Answer from the drawing. Dimensions are ordinates in mm from the lowest x, y and z of the part. A direction names the side the tool comes from. Give positions to 0.01 mm unless a question says otherwise; leave off trailing zeros. Order: outer loops, then holes, each group sorted by start corner. A loop starts at its lowest first (then second) coordinate and runs counter-clockwise, first axis right, second up.
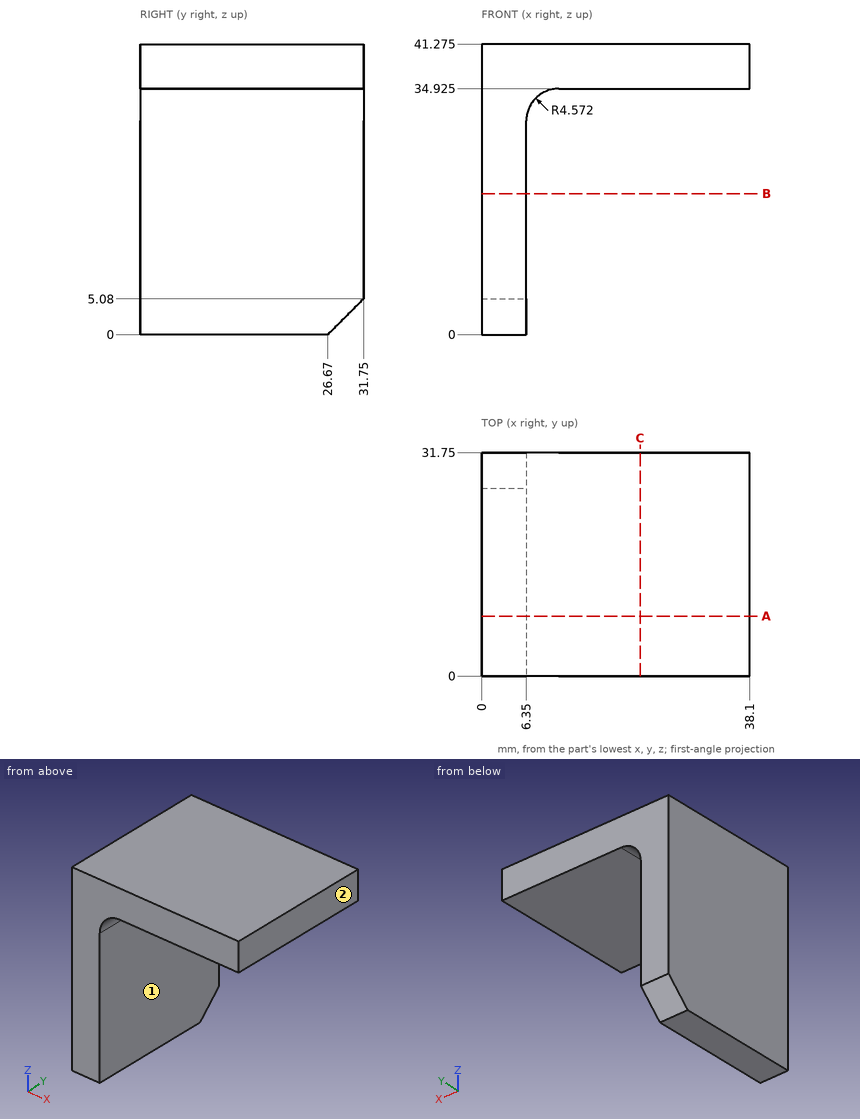
1. Given P1, Ø3, axis at x = 10.5, y = 21.5, coming from the -Z side; P2, Ø10, axis at x = 29.5, y = 11, coming from the -Z side (3 decimals); P3, Ø3, axis at y = 22, z = 23.5, coming from the +X side, each flat-ended and moving along its own axis, determine where each tip first touches the part or whether it passes through.
Findings below:
P1: stops at z = 34.5
P2: stops at z = 34.925
P3: stops at x = 6.35
2. The part is cut by section C-C (x = 22.5). Write down the section's boundary in (y, z) (3 decimals), then the cut area to 3 significant figures.
Findings below:
outline: (0, 34.925) - (31.75, 34.925) - (31.75, 41.275) - (0, 41.275) - close
area: 202 mm2
3. Which of the six approach directions +Z, -Z, +X, -X, +Y, -Y give full straight-line access (tool end or side, diameter ignored) to the marked faces 1 and 2?
Findings below:
face 1: -Z, +X, +Y, -Y
face 2: +Z, -Z, +X, +Y, -Y
4. Straight lines are drawn through the part: probe 1 along Z at (x, y) = (15.5, 7.5) (3 decimals); probe 2 along X at (y, z) = (17, 26.5). For each, find the intervals that lie inside material, in ascending order.
Findings below:
probe 1: z = 34.925 to 41.275
probe 2: x = 0 to 6.35
5. The part is cut by section A-A (y = 8.5). Write down the section's boundary in (x, z) (3 decimals).
Findings below:
outline: (0, 0) - (6.35, 0) - (6.35, 30.353) arc R4.572 cw to (10.922, 34.925) - (38.1, 34.925) - (38.1, 41.275) - (0, 41.275) - close
6. The part is cut by section B-B (z = 20). Write down the section's boundary in (x, y).
Findings below:
outline: (0, 0) - (6.35, 0) - (6.35, 31.75) - (0, 31.75) - close
